```python
from build123d import *

# Parameters (mm, degrees)
F0_R     = 1.5
F1_DEPTH = 10
F2_R     = 2.8
F3_DEPTH = 3
F5_DEPTH = 1.5
F6_SIZE  = 0.25


with BuildPart() as f1:
    # F0 (on Top) → F1 (new body)
    with BuildSketch(Plane.XY):
        Circle(F0_R)
    extrude(amount=F1_DEPTH)

    # F2 (on Top) → F3 (join)
    with BuildSketch(Plane.XY):
        Circle(F2_R)
    extrude(amount=-F3_DEPTH)

    # F4 (on face) → F5 (cut)
    with BuildSketch(Plane(origin=(0, 0, -3), x_dir=(1, 0, 0), z_dir=(0, 0, -1))):
        Polygon((0.446582, -1.372552), (1.411956, -0.299524), (0.965373, 1.073027), (-0.446582, 1.372552), (-1.411956, 0.299524), (-0.965373, -1.073027), align=None)
    extrude(amount=-F5_DEPTH, mode=Mode.SUBTRACT)

    # F6
    f6_edges = [f1.edges().sort_by_distance(p)[0] for p in [
        (-2.8, 0, -3),
        (-1.5, 0, 10),
        (-2.8, 0, 0),
    ]]
    chamfer(f6_edges, length=F6_SIZE)


solid = f1.part
```
The model under review builds one solid part; all positions refer to its coordinate system, in mm. A direction names the side the tool comes from. Round coordinates to 2 decimals unless told otherwise and drop trailing zeros. Loops run counter-clockwise (first coordinate to the right, second up) from the corner with the lowest first, then second, coordinate; pieces in that order, holes last. Notation, with made-up numbers: (78.25, 20) - (89.25, 20) arc R20 cw to (89.25, 47) - close; hole circle Ø10 at (46.25, 1.5). An arc over 180 degrees is marked (long way). Write each question's results on one line, items separated by ' | '. Start each with the question number.
Q1. Take a section at C-C on z = 5.25. Give the boundary of the cut face in (x, y), plus the area to 3 significant figures.
Q2. Take a section at A-A on y = 0. Give the boundary of the cut face in (x, z), plus the area to 3 significant figures.
Q3. Insertion check: P1, Ø1.5, axis at x = -1, z = 2.5, coming from the +Y side; P2, Ø0.8, axis at x = -0.5, y = 0, coming from the -Z side. Each pin has a flat end and moves straight along its axis. Give the tip position at first contact, or say it passes through.
Q4. Wall thickness on line 1 along Z through (x, y) = (1.25, 1.05); line 2 along Z through (x, y) = (1.1, 0.45); line 3 along X through (y, z) = (0.6, 3.5): over which ranges is each line inside the solid? List them lowest first. Write a range as [from, to].
Q5. Take a section at B-B on x = 0. Give the boundary of the cut face in (y, z).
Q6. Draft analysis for pull direction Y (two halves, no side actions). For faces 4 (the flat face through (1.19, -0.38, -2.26)), 5 (the cylindrical face through (-2.8, 0.1, -1.5)), 6 (the flat face through (0, -2, 0)), 7 (the flat face through (-1.19, 0.38, -2.26)), state which applies: pulls with the +Y half, pulls with the -Y half, needs draft (parallel to the pull), parting line crosses it, or undercut.
Q7. Tool access review of faces 1 (the flat face through (0.923, 0.844, -2.26)), 2 (the cylindrical face through (-1.5, 0.07, 4.81)), 3 (the flat face through (0, 0, 10)): name each direction out of +Z, -Z, +X, -X, +Y, -Y from which nothing blocks a thin tool from reaching the whole face with its end or side.
Data:
1) outline: circle Ø3 at (0, 0) | area: 7.07 mm²
2) outline: (-2.8, -2.75) - (-2.55, -3) - (-1.31, -3) - (-1.31, -1.5) - (1.31, -1.5) - (1.31, -3) - (2.55, -3) - (2.8, -2.75) - (2.8, -0.25) - (2.55, 0) - (1.5, 0) - (1.5, 9.75) - (1.25, 10) - (-1.25, 10) - (-1.5, 9.75) - (-1.5, 0) - (-2.55, 0) - (-2.8, -0.25) - close | area: 42.7 mm²
3) P1: stops at y = 1.48 | P2: stops at z = -1.5
4) line 1: z = [-3, 0] | line 2: z = [-1.5, 10] | line 3: x = [-1.37, 1.37]
5) outline: (-2.8, -2.75) - (-2.55, -3) - (-1.28, -3) - (-1.28, -1.5) - (1.28, -1.5) - (1.28, -3) - (2.55, -3) - (2.8, -2.75) - (2.8, -0.25) - (2.55, 0) - (1.5, 0) - (1.5, 9.75) - (1.25, 10) - (-1.25, 10) - (-1.5, 9.75) - (-1.5, 0) - (-2.55, 0) - (-2.8, -0.25) - close
6) face 4: undercut | face 5: parting line crosses it | face 6: needs draft | face 7: undercut
7) face 1: -Z | face 2: +Z | face 3: +Z, +X, -X, +Y, -Y
